Autodesk Inventor part; units mm, degrees
ref_plane "YZ Plane" through (0, 0, 0) normal (1, 0, 0) x (0, 1, 0)
ref_plane "XZ Plane" through (0, 0, 0) normal (0, 1, 0) x (-1, 0, 0)
ref_plane "XY Plane" through (0, 0, 0) normal (0, 0, 1) x (1, 0, 0)
sketch "Sketch1" plane through (0, 0, 0) normal (0, 1, 0) x (-1, 0, 0)
  line L0 (0, 0) -> (10, 0)
  line L1 (10, 0) -> (10, -10)
  line L2 (10, -10) -> (0, -10)
  line L3 (0, -10) -> (0, 0)
  line L4 (70, -10) -> (60, -10)
  line L5 (60, -10) -> (60, 0)
  line L6 (60, 0) -> (70, 0)
  line L7 (70, 0) -> (70, -10)
  line L8 (70, -70) -> (60, -70)
  line L9 (60, -70) -> (60, -60)
  line L10 (60, -60) -> (70, -60)
  line L11 (70, -60) -> (70, -70)
  line L12 (10, -70) -> (0, -70)
  line L13 (0, -70) -> (0, -60)
  line L14 (0, -60) -> (10, -60)
  line L15 (10, -60) -> (10, -70)
  dimension "d0" = 10
  dimension "d1" = 10
  dimension "d2" = 10
  dimension "d3" = 10
  dimension "d4" = 10
  dimension "d5" = 10
  dimension "d6" = 10
  dimension "d7" = 10
  dimension "d8" = 50
  dimension "d9" = 50
extrude "Extrusion1" add sketch "Sketch1" along normal blind 127
sketch "Sketch2" plane through (-70, 0, 0) normal (0, 0, 1) x (1, 0, 0)
  line L0 (10, 0) -> (10, 127) construction
  line L1 (10, 0) -> (60, 50)
  line L2 (60, 0) -> (60, 127) construction
  line L3 (10, 0) -> (80.7107, 0) construction
  line L4 (10, 10) -> (60, 60)
  line L5 (60, 60) -> (10, 110)
  line L6 (60, 60) -> (130.7107, 60) construction
  line L7 (10, 120) -> (60, 70)
  line L8 (60, 70) -> (60, 50)
  line L9 (10, 120) -> (10, 110)
  line L10 (10, 0) -> (10, 10)
  point P0 (70, 0)
  dimension "d12" = 45
  dimension "d14" = 10
  dimension "d15" = 135
  dimension "d16" = 10
  dimension "d17" = 10
extrude "Extrusion2" add sketch "Sketch2" against normal blind 10
sketch "Sketch3" plane through (0, 0, 0) normal (1, 0, 0) x (0, 0, -1)
  line L0 (10, 0) -> (10, 127) construction
  line L1 (10, 0) -> (60, 50)
  line L2 (10, 0) -> (70, 0) construction
  line L3 (60, 0) -> (60, 127) construction
  line L4 (60, 0) -> (70, 0) construction
  line L5 (60, 127) -> (60, 0)
  line L6 (10, 10) -> (60, 60)
  line L7 (10, 0) -> (10, 127)
  line L8 (60, 60) -> (10, 110)
  line L9 (60, 60) -> (70, 60) construction
  line L10 (10, 120) -> (60, 70)
  dimension "d20" = 45
  dimension "d21" = 10
  dimension "d22" = 135
  dimension "d23" = 10
extrude "Extrusion3" add sketch "Sketch3" against normal blind 10 contours L7 L6 L5 L1 | L8 L7 L10 L5
sketch "Sketch4" plane through (0, 0, -70) normal (0, 0, -1) x (-1, 0, 0)
  line L0 (10, 0) -> (10, 127) construction
  line L1 (10, 0) -> (60, 50)
  line L2 (60, 10) -> (60, 110) construction
  line L3 (10, 0) -> (80.7107, 0) construction
  line L4 (10, 10) -> (60, 60)
  line L5 (60, 120) -> (60, 127) construction
  line L6 (60, 127) -> (60, 0)
  line L7 (10, 0) -> (10, 127)
  line L8 (60, 60) -> (10, 110)
  line L9 (60, 60) -> (70, 60) construction
  line L10 (10, 120) -> (60, 70)
  point P0 (70, 0)
  point P1 (60, 60)
  point P2 (60, 60)
  point P3 (60, 50)
  dimension "d26" = 45
  dimension "d27" = 10
  dimension "d28" = 135
  dimension "d29" = 10
extrude "Extrusion4" add sketch "Sketch4" against normal blind 10 contours L7 L4 L6 L1 | L8 L7 L10 L6
sketch "Sketch5" plane through (-70, 0, -70) normal (-1, 0, 0) x (0, 0, 1)
  line L0 (10, 0) -> (10, 127) construction
  line L1 (60, 10) -> (60, 50) construction
  line L2 (10, 0) -> (60, 50)
  line L3 (10, 0) -> (80.7107, 0) construction
  line L4 (10, 127) -> (10, 0)
  line L5 (60, 127) -> (60, 0)
  line L6 (10, 10) -> (60, 60)
  line L7 (60, 60) -> (10, 110)
  line L8 (60, 60) -> (70, 60) construction
  line L9 (60, 70) -> (10, 120)
  line L10 (10, 70) -> (60, 120) construction
  point P0 (70, 0)
  dimension "d32" = 45
  dimension "d33" = 135
  dimension "d34" = 10
  dimension "d35" = 10
extrude "Extrusion5" add sketch "Sketch5" against normal blind 10 contours L4 L6 L5 L2 | L7 L4 L9 L5
sketch "Sketch6" plane through (0, 0, 0) normal (0, -1, 0) x (1, 0, 0)
  line L0 (-70, -10) -> (-70, 0) construction
  line L1 (0, -70) -> (-70, -70)
  line L2 (-70, -70) -> (-70, 0)
  line L3 (-70, 0) -> (0, 0)
  line L4 (0, 0) -> (0, -70)
  point P0 (0, 0)
extrude "Extrusion6" add sketch "Sketch6" along normal blind 2.5
properties part number "TRUSSTEST"
Could you check a few things on this model? Use its own coordinates, in mm. A direction names the side the tool comes from. Coordinates: 2 decimals unless noted, no trailing zeros. Order: outer loops, then holes, each group sorted by start corner. A loop starts at its lowest first (then second) coordinate and runs counter-clockwise, first axis right, second up. Notation, with made-up numbers: (-33, 46.25) - (-6, 46.25) arc R24 cw to (-6, 72.25) - close; hole circle Ø10 at (-7.75, 10). An arc over 180 degrees is marked (long way). Answer in a Markdown table with one row per item. Add a question column.
(1) If we section it at D-D, the plane z = -6.5: Please give me the cut outline in (x, y).
(2) I need wall thicknesses on L1, parallel to Z at x = -64, y = 16; L2, parallel to Y at x = -46.5, z = -61; L3, parallel to X at y = 89, z = -5.5. Which ranges of each line are inside material? Lowest first, please.
(3) If we section it at B-B, the plane y = 107: State how many separate pieces and enclosed holes the cut face has, then the cut area to 3 significant figures.
(4) If we section it at A-A, the plane z = -54: Please give me the cut outline in (x, y), then the cut area to 3 significant figures.
(5) If we section it at C-C, the plane x = -8: Please give me the cut outline in (y, z), then the cut area to 4 significant figures.
(6) Will these pins go through, and if not, where does the flat tip stop? pin 1 (6 mm diameter, centred on x = -40.5, y = 11.5, fed in from +Z); pin 2 (2 mm diameter, centred on x = -65.5, y = 125, fed in from +Z); pin 3 (1.5 mm diameter, centred on x = -36, z = -19.5, fed in from +Y); pin 4 (12 mm diameter, centred on x = -59, z = -37.5, fed in from +Y).
(7) On a 3-axis mill with a long thin cutter (end or side, diameter ignored), from which of +Z, -Z, +X, -X, +Y, -Y can I reach the whole of each face in a straight line? I mean faces 1 (the face through (-10, 123, -65)), 2 (the face through (-35, 0, -35)), 3 (the face through (-65, 127, -5)). Say none if no direction works.
(8) If we mould it in two halves opening along Z, with no side actions, what happens to faces 4 (the face through (-50, 72, -70)), 5 (the face through (-10, 77, -45)), 6 (the face through (-25, 77, -10))? For each: released by +Z, released by -Z, zero draft, split by the parting line, or undercut.
Results are:
| question | item | result |
|---|---|---|
| 1 | outline | (-70, -2.5) - (0, -2.5) - (0, 127) - (-10, 127) - (-10, 70) - (-60, 120) - (-60, 127) - (-70, 127) - close; hole (-60, 0) - (-10, 0) - (-10, 50) - close; hole (-60, 10) - (-10, 60) - (-60, 110) - close |
| 2 | L1 | z = -70 to -60, -54 to -44, -10 to 0 |
| 2 | L2 | y = -2.5 to 0, 36.5 to 46.5, 73.5 to 83.5 |
| 2 | L3 | x = -70 to -60, -39 to -29, -10 to 0 |
| 3 | separate pieces | 8 |
| 3 | enclosed holes | 0 |
| 3 | area | 800 mm2 |
| 4 | outline | (-70, -2.5) - (0, -2.5) - (0, 0) - (-70, 0) - close; (-70, 6) - (-60, 6) - (-60, 16) - (-70, 16) - close; (-70, 104) - (-60, 104) - (-60, 114) - (-70, 114) - close; (-10, 44) - (0, 44) - (0, 54) - (-10, 54) - close; (-10, 66) - (0, 66) - (0, 76) - (-10, 76) - close |
| 4 | area | 575 mm2 |
| 5 | outline | (-2.5, -70) - (127, -70) - (127, -60) - (70, -60) - (120, -10) - (127, -10) - (127, 0) - (-2.5, 0) - close; hole (0, -60) - (50, -60) - (0, -10) - close; hole (10, -10) - (60, -60) - (110, -10) - close |
| 5 | area | 3,715 mm2 |
| 6 | pin 1 | passes through |
| 6 | pin 2 | stops at z = 0 |
| 6 | pin 3 | stops at y = 0 |
| 6 | pin 4 | stops at y = 103.42 |
| 7 | face 1 | +Z, -Z, +Y |
| 7 | face 2 | none |
| 7 | face 3 | +Z, -Z, +X, -X, +Y |
| 8 | face 4 | released by -Z |
| 8 | face 5 | zero draft |
| 8 | face 6 | undercut |
